Input: dimensioned drawing with shaded views. Units: mm. Origin: part minimum x, y, z. A direction names the side the tool comes from. Coordinates: 2 decimals unless noted, no trailing zeros. Order: outer loops, then holes, each group sorted by start corner. A loop starts at its lowest first (then second) coordinate and runs counter-clockwise, first axis right, second up.
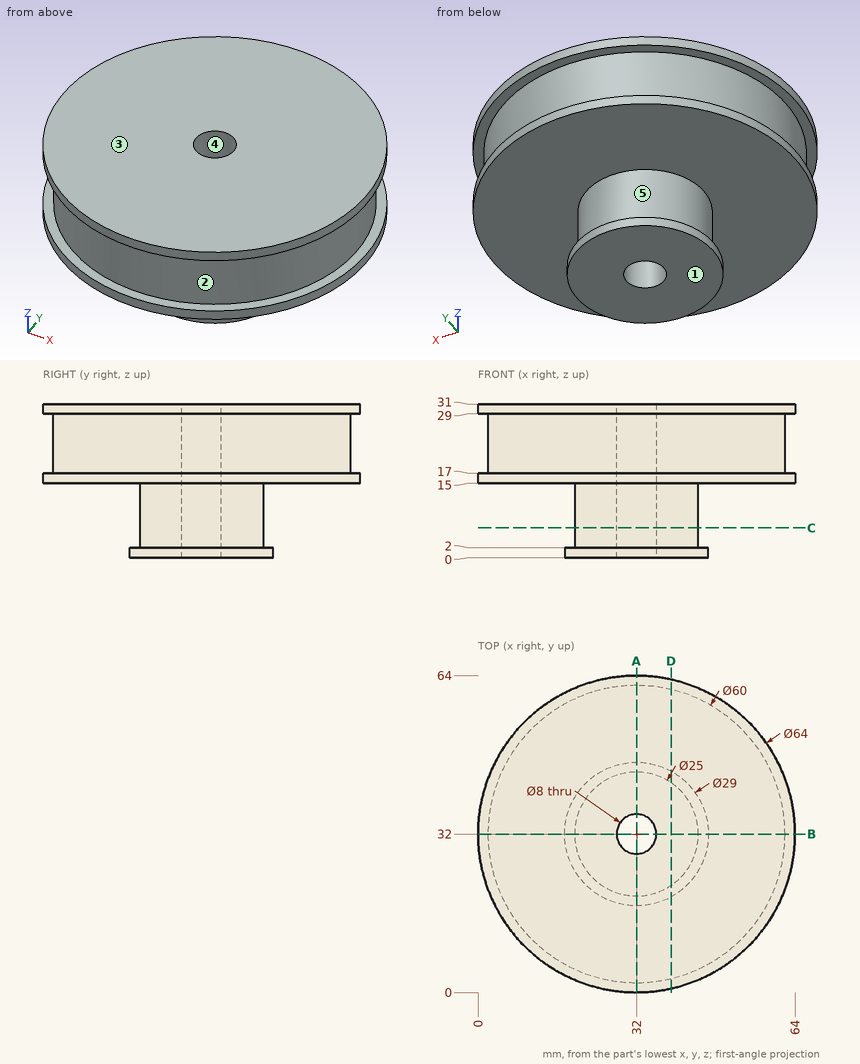
1. Section query D-D on x = 39. Return loops of the section in (y, z).
Findings:
outline: (0.78, 15) - (21.64, 15) - (21.64, 2) - (19.3, 2) - (19.3, 0) - (44.7, 0) - (44.7, 2) - (42.36, 2) - (42.36, 15) - (63.22, 15) - (63.22, 17) - (61.17, 17) - (61.17, 29) - (63.22, 29) - (63.22, 31) - (0.78, 31) - (0.78, 29) - (2.83, 29) - (2.83, 17) - (0.78, 17) - close
2. Access query for the marked faces 1 and 2. Directions: +Z, -Z, +X, -X, +Y, -Y. A direction counts if a zero-diameter tool reaches every point of the face in a straight line with its end or side. Return the directions, or none.
Findings:
face 1: -Z, +X, -X, +Y, -Y
face 2: none
3. Pin query (flat end, axial travel): P1, Ø5, axis at x = 22, y = 48.5, coming from the -Z side; P2, Ø8, axis at y = 42, z = 5, coming from the -X side; P3, Ø1, axis at y = 25, z = 24.5, coming from the +X side. Return the tip coordinate at first contact, or that it passes through.
Findings:
P1: stops at z = 15
P2: stops at x = 19.5
P3: stops at x = 61.29
4. Draft query along X for the marked faces 3, 4 and 5. Return one class per face: released by +X, released by -X, zero draft, split by the parting line, or undercut.
Findings:
face 3: zero draft
face 4: undercut
face 5: split by the parting line
5. Ray query, line 1 (Z direction, x = 41, y = 61.5); line 2 (Y direction, x = 32, z = 21); line 3 (Z direction, x = 58, y = 21). Return the intervals inside material, ascending.
Findings:
line 1: z = 15 to 17, 29 to 31
line 2: y = 2 to 28, 36 to 62
line 3: z = 15 to 31
6. Section query C-C on z = 6. Return loops of the section in (x, y), plus the area to 3 significant figures.
Findings:
outline: circle Ø25 at (32, 32); hole circle Ø8 at (32, 32)
area: 441 mm2
7. Section query A-A on x = 32. Return loops of the section in (y, z), plus the area to 3 significant figures.
Findings:
outline: (0, 15) - (19.5, 15) - (19.5, 2) - (17.5, 2) - (17.5, 0) - (28, 0) - (28, 31) - (0, 31) - (0, 29) - (2, 29) - (2, 17) - (0, 17) - close; (36, 0) - (46.5, 0) - (46.5, 2) - (44.5, 2) - (44.5, 15) - (64, 15) - (64, 17) - (62, 17) - (62, 29) - (64, 29) - (64, 31) - (36, 31) - close
area: 1,110 mm2
